from build123d import *

# Parameters (mm, degrees)
SKETCH1_W           = 69.85
SKETCH1_H           = 55.118
SKETCH1_R           = 1.98755
SKETCH1_R_2         = 2.54
SKETCH1_W_2         = 40.386
SKETCH1_H_2         = 20.828
BOSS_EXTRUDE1_DEPTH = 3.048


with BuildPart() as part:
    # Sketch1 → Boss-Extrude1 (new body)
    with BuildSketch(Plane(origin=(0, 0, 0), x_dir=(1, 0, 0), z_dir=(0, 1, 0))):
        with Locations((0, 13.335)):
            Rectangle(SKETCH1_W, SKETCH1_H)
        with Locations((-25.0571, -5.5499)):
            Circle(SKETCH1_R, mode=Mode.SUBTRACT)
        with Locations((-25.0571, 5.5499)):
            Circle(SKETCH1_R, mode=Mode.SUBTRACT)
        with Locations((25.0571, -5.5499)):
            Circle(SKETCH1_R, mode=Mode.SUBTRACT)
        with Locations((25.0571, 5.5499)):
            Circle(SKETCH1_R, mode=Mode.SUBTRACT)
        with Locations((-26.67, 36.1315)):
            Circle(SKETCH1_R_2, mode=Mode.SUBTRACT)
        with Locations((-26.67, 26.6065)):
            Circle(SKETCH1_R_2, mode=Mode.SUBTRACT)
        with Locations((26.67, 26.6065)):
            Circle(SKETCH1_R_2, mode=Mode.SUBTRACT)
        with Locations((26.67, 36.1315)):
            Circle(SKETCH1_R_2, mode=Mode.SUBTRACT)
        Rectangle(SKETCH1_W_2, SKETCH1_H_2, mode=Mode.SUBTRACT)
    extrude(amount=BOSS_EXTRUDE1_DEPTH)


solid = part.part
Input: part model. Units: mm. Frame: model coordinates. A direction names the side the tool comes from. Give positions to 0.01 mm unless a question says otherwise; leave off trailing zeros. Write each loop counter-clockwise with the first axis right and the second up, starting at its lowest first coordinate (ties: lowest second). Pieces come first, ordered by that corner, then holes.
Q1. Material intervals for probe 1 along X at (y, z) = (1.2, -5.5) (3 decimals); probe 2 along X at (y, z) = (0.7, 1) (3 decimals); probe 3 along X at (y, z) = (1.8, -4) (3 decimals), sorted ascending.
Q2. Section B-B, the plane z = -25. Output: boundary loops of the cut face in (x, y) (3 decimals), plus the area to 3 significant figures.
Q3. Set-up query: faces 5 (the face through (0, 2, 10.414)), 6 (the face through (0, 3.048, -20)). Return all of +Z, -Z, +X, -X, +Y, -Y with unobstructed straight access to the full face (end or side cutting, diameter ignored); none if empty.
Q4. Section C-C, the plane y = 2.1. State how many separate pieces and enclosed holes the cut face has, plus the area to 3 significant figures.
Q5. Pull-direction query (X, two-part tool) for faces 1 (the face through (-34.925, 2, -13)), 2 (the face through (0, 2, 14.224)), 3 (the face through (20.193, 2, 0)), 4 (the face through (-26.6, 1.5, 6.8)); classes: pulls with the +X half, pulls with the -X half, needs draft (parallel to the pull), parting line crosses it, or undercut.
Q6. First-contact query: P1, Ø2, axis at x = 21, z = 4.5, coming from the -Y side. Flat tip, straight axial feed; report the tip coordinate or a pass-through.
Q7. Section A-A, the plane x = -2.5. Output: boundary loops of the cut face in (y, z).
Filled in:
1. probe 1: x = -34.925 to -27.044, -23.07 to -20.193, 20.193 to 23.07, 27.044 to 34.925
1. probe 2: x = -34.925 to -20.193, 20.193 to 34.925
1. probe 3: x = -34.925 to -26.301, -23.813 to -20.193, 20.193 to 23.813, 26.301 to 34.925
2. outline: (-34.925, 0) - (-28.637, 0) - (-28.637, 3.048) - (-34.925, 3.048) - close; (-24.703, 0) - (24.703, 0) - (24.703, 3.048) - (-24.703, 3.048) - close; (28.637, 0) - (34.925, 0) - (34.925, 3.048) - (28.637, 3.048) - close
2. area: 189 mm2
3. face 5: +Y, -Y
3. face 6: +Z, -Z, +X, -X, +Y
4. separate pieces: 1
4. enclosed holes: 9
4. area: 2,880 mm2
5. face 1: pulls with the -X half
5. face 2: needs draft
5. face 3: undercut
5. face 4: undercut
6. P1: stops at y = 0
7. outline: (0, -40.89) - (3.05, -40.89) - (3.05, -10.41) - (0, -10.41) - close; (0, 10.41) - (3.05, 10.41) - (3.05, 14.22) - (0, 14.22) - close
